For this review, take the finished solid that the model builds, in its own axes (mm). A direction names the side the tool comes from. Give positions to 0.01 mm unless a question says otherwise; leave off trailing zeros. Loops run counter-clockwise (first coordinate to the right, second up) from the corner with the lowest first, then second, coordinate; pieces in that order, holes last.
Autodesk Inventor part; units mm, degrees
ref_plane "YZ Plane" through (0, 0, 0) normal (1, 0, 0) x (0, 1, 0)
ref_plane "XZ Plane" through (0, 0, 0) normal (0, 1, 0) x (-1, 0, 0)
ref_plane "XY Plane" through (0, 0, 0) normal (0, 0, 1) x (1, 0, 0)
sketch "スケッチ1" plane through (0, 0, 0) normal (0, 0, 1) x (1, 0, 0)
  circle A0 centre (0, 0) radius 2
  dimension "d1" = 4
extrude "押し出し1" add sketch "スケッチ1" along normal blind 8
sketch "スケッチ2" plane through (0, 0, 0) normal (0, 0, -1) x (-1, 0, 0)
  circle A0 centre (0, 0) radius 2
  circle A1 centre (0, 0) radius 4
  dimension "d4" = 8
extrude "押し出し2" add sketch "スケッチ2" along normal blind 3.1 contours A0 | A1
fillet "フィレット1" radius 3.1 1 edges at (4, 0, -3.1)
thread "ねじ1"
properties part number "ネジ鍋m4,08" material "鋼、高強度、低合金"
Q1. Consider section A-A on z = 7.5. Give the boundary of the cut face in (x, y).
Answers:
outline: circle Ø4 at (0, 0)
Q2. For probe 1 along Z at (x, y) = (0, 1); probe 2 along Y at (x, z) = (1.75, 6); probe 3 along X at (y, z) = (-1.25, 5.25), list the stretches that pass through material, from the lowest coordinate up.
Answers:
probe 1: z = -3.1 to 8
probe 2: y = -0.97 to 0.97
probe 3: x = -1.56 to 1.56
Q3. Machinability: for faces 1 (the flat face through (2, -1, 0)), 2 (the flat face through (0, 0, -3.1)), which of the approach directions +Z, -Z, +X, -X, +Y, -Y give a long, thin tool a straight path to every point of the face, cutting with its end or side? Answer none if there is none.
Answers:
face 1: +Z
face 2: -Z, +X, -X, +Y, -Y
Q4. Mouldability with a two-part tool opening along X and no side actions: class faces 3 (the flat face through (0, 0, 8)), 4 (the cylindrical face through (0, 2, 4)) as +X half, -X half, draft (parallel to the pull), parting line (faces both ways), or undercut.
Answers:
face 3: draft
face 4: parting line
Q5. For pin 1 Ø2 at (x, y) = (1, 2.5) entering from -Z; pin 2 Ø1 at (y, z) = (-1, 6) entering from +X; pin 3 Ø4 at (x, z) = (2, 4) entering from -Y, all flat-tipped, find the tip position at first contact; note any pin that passes through.
Answers:
pin 1: stops at z = -3
pin 2: stops at x = 1.94
pin 3: stops at y = -2
